Geometry check sheet. Reference: the model listing, model coordinates, mm. Give positions to 0.01 mm unless a question says otherwise; leave off trailing zeros. Order: outer loops, then holes, each group sorted by start corner. A loop starts at its lowest first (then second) coordinate and runs counter-clockwise, first axis right, second up.
from build123d import *

# Parameters (mm, degrees)
SKETCH1_W                   = 15
SKETCH1_H                   = 15
BOSS_EXTRUDE1_DEPTH         = 8
TAP_DRILL_FOR_M5X0_8_TAP1_D = 4.2
F_5_0_5_DIAMETER_HOLE1_D    = 5


with BuildPart() as part:
    # Sketch1 → Boss-Extrude1 (new body)
    with BuildSketch(Plane.XY):
        with Locations((7.5, 7.5)):
            Rectangle(SKETCH1_W, SKETCH1_H)
    extrude(amount=BOSS_EXTRUDE1_DEPTH)

    # Tap Drill for M5x0.8 Tap1 (through all)
    with Locations(Plane.XY.offset(8)):
        with Locations((10.5, 10.5)):
            Hole(TAP_DRILL_FOR_M5X0_8_TAP1_D / 2)

    # Ø5.0 (5) Diameter Hole1 (through all)
    with Locations(Plane.ZY):
        with Locations((4, 4.5)):
            Hole(F_5_0_5_DIAMETER_HOLE1_D / 2)


solid = part.part
Item 1: Scan lines: L1, parallel to Y at x = 10, z = 3.5; L2, parallel to Y at x = 7.75, z = 4; L3, parallel to X at y = 10.25, z = 5. Record each from-to range of solid material in increasing order.
Reported:
L1: y = 0 to 2.05, 6.95 to 8.46, 12.54 to 15
L2: y = 0 to 2, 7 to 15
L3: x = 0 to 8.41, 12.59 to 15
Item 2: Sectioned sample at D-D (y = 4.5). Enter the section's corners in (x, z), and give its area (3 significant figures).
Reported:
outline: (0, 0) - (15, 0) - (15, 1.5) - (0, 1.5) - close; (0, 6.5) - (15, 6.5) - (15, 8) - (0, 8) - close
area: 45.0 mm2
Item 3: Sectioned sample at A-A (z = 6). Enter the section's corners in (x, y), and give its area (3 significant figures).
Reported:
outline: (0, 0) - (15, 0) - (15, 3) - (0, 3) - close; (0, 6) - (15, 6) - (15, 15) - (0, 15) - close; hole circle Ø4.2 at (10.5, 10.5)
area: 166 mm2
Item 4: Draft check along Y on faces 1 (the flat face through (7, 0, 4)), 2 (the flat face through (7, 8, 0)), 3 (the cylindrical face through (12.6, 10.59, 3.94)). Enter one of: released by +Y, released by -Y, zero draft, split by the parting line, or undercut.
Reported:
face 1: released by -Y
face 2: zero draft
face 3: undercut
Item 5: Sectioned sample at B-B (x = 10.5). Enter the section's corners in (y, z), and give its area (3 significant figures).
Reported:
outline: (0, 0) - (8.4, 0) - (8.4, 8) - (0, 8) - close; (12.6, 0) - (15, 0) - (15, 8) - (12.6, 8) - close; hole circle Ø5 at (4.5, 4)
area: 66.8 mm2
Item 6: Sectioned sample at C-C (y = 3). Enter the section's corners in (x, z).
Reported:
outline: (0, 0) - (15, 0) - (15, 2) - (0, 2) - close; (0, 6) - (15, 6) - (15, 8) - (0, 8) - close
